from build123d import *

# Parameters (mm, degrees)
SKETCH5_R          = 10
CUT_EXTRUDE1_DEPTH = 4


with BuildPart() as part:
    # Sketch1 → Revolve1 (revolve)
    with BuildSketch(Plane.XY, mode=Mode.PRIVATE) as revolve1_sk:
        Polygon((-25, 89), (-35, 89), (-35, 84), (-30, 84), (-30, 79), (-35, 79), (-35, 74), (-30, 74), (-30, 43), (-42.976744186, 12), (-72.5, 12), (-72.5, 0), (-43, 0), (-25, 43), align=None)
    revolve(revolve1_sk.sketch.rotate(Axis((0, 0, 0), (0, 1, 0)), 180), axis=Axis((0, 0, 0), (0, 1, 0)))

    # Sketch5 → Cut-Extrude1 (cut)
    with BuildSketch(Plane(origin=(0, 12, 0), x_dir=(1, 0, 0), z_dir=(0, 1, 0))):
        with Locations(Location((0, 58.5, 0), (0, 0, 180))):
            Circle(SKETCH5_R)
        with Locations(Location((58.5, 0, 0), (0, 0, 180))):
            Circle(SKETCH5_R)
        with Locations(Location((0, -58.5, 0), (0, 0, 180))):
            Circle(SKETCH5_R)
        with Locations(Location((-58.5, 0, 0), (0, 0, 180))):
            Circle(SKETCH5_R)
    extrude(amount=-CUT_EXTRUDE1_DEPTH, mode=Mode.SUBTRACT)


solid = part.part
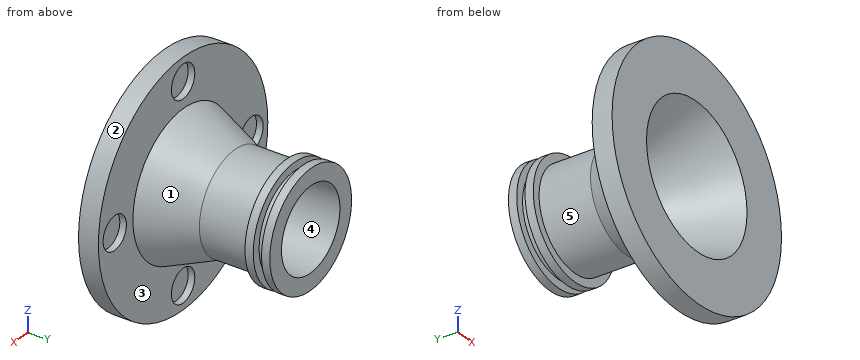
The model under review builds one solid part; all positions refer to its coordinate system, in mm. Face numbers are marked on the shaded views. A direction names the side the tool comes from. Coordinates: 2 decimals unless noted, no trailing zeros. Loops run counter-clockwise (first coordinate to the right, second up) from the corner with the lowest first, then second, coordinate; pieces in that order, holes last. Notation, with made-up numbers: M 3,29 L 43,29 A16 ccw 43,41 Z; hole C 30.25,33 d3. An arc over 180 degrees is marked long. Put each result on its own line as item: value. Start each with the question number.
Q1. The part is to be moulded in two halves that separate along Y. For the marked faces 3, 4 and 5, say which applies: +Y half, -Y half, draft (parallel to the pull), parting line (faces both ways), or undercut.
Q2. Clearance check with flat-ended pins moving along their axes: pin 1 (12 mm diameter, centred on x = -53.5, y = 12, fed in from -Z); pin 2 (22 mm diameter, centred on x = 55, z = -4, fed in from +Y); pin 3 (5 mm diameter, centred on x = 12.5, y = 22, fed in from -Z); pin 4 (1 mm diameter, centred on x = 36.5, y = 75.5, fed in from +Z). State where each tip first meets the part, or that it passes through.
Q3. Add section D-D (y = 39). Write out the cut boundary in (x, z).
Q4. Add section A-A (y = 51). Write out the cut boundary in (x, z), and give its area (3 significant figures).
Q5. Wall thickness on line 1 (Y direction, x = 23.5, z = 40); line 2 (Z direction, x = 0, y = 10.15); line 3 (Z direction, x = -6, y = 30.5): over which ranges is each line inside the solid? List them lowest first.
Q6. For the marked faces 1 and 2, list the 3-axis set-ups (+Z, -Z, +X, -X, +Y, -Y) from which the entire face can be reached by the end or side of a thin tool; tool diameter is ignored.
Q7. Add section C-C (x = -58.5). Write out the cut boundary in (y, z), and give its area (3 significant figures).
Q8. Add section B-B (z = -58.5). Write out the cut boundary in (x, y).
Answers:
1. face 3: +Y half
1. face 4: draft
1. face 5: undercut
2. pin 1: stops at z = -54.77
2. pin 2: stops at y = 12
2. pin 3: stops at z = -38.07
2. pin 4: passes through
3. outline: C 0,0 d63.35; hole C 0,0 d53.35
4. outline: C 0,0 d60; hole C 0,0 d50
4. area: 864 mm^2
5. line 1: y = 0 to 12
5. line 2: z = -72.5 to -68.5, -48.5 to -38.75, 38.75 to 48.5, 68.5 to 72.5
5. line 3: z = -34.72 to -29.63, 29.63 to 34.72
6. face 1: none
6. face 2: +Y, -Y
7. outline: M 0,-42.83 L 12,-42.83 L 12,-10 L 8,-10 L 8,10 L 12,10 L 12,42.83 L 0,42.83 Z
7. area: 948 mm^2
8. outline: M -42.83,0 L 42.83,0 L 42.83,12 L 10,12 L 10,8 L -10,8 L -10,12 L -42.83,12 Z
